Autodesk Inventor part; units mm, degrees
ref_plane "Work Plane1" through (75.8893, 0, 0) normal (0, 0.8660254, -0.5) x (-1, 0, 0)
ref_plane "YZ Plane" through (0, 0, 0) normal (1, 0, 0) x (0, 1, 0)
ref_plane "XZ Plane" through (0, 0, 0) normal (0, 1, 0) x (-1, 0, 0)
sketch "Sketch1" plane through (0, 0, 0) normal (1, 0, 0) x (0, 1, 0)
  line L0 (26.5724, 0) -> (13.2862, -23.0124)
  line L1 (13.2862, -23.0124) -> (-13.2862, -23.0124)
  line L2 (-13.2862, -23.0124) -> (-26.5724, 0)
  line L3 (-26.5724, 0) -> (-13.2862, 23.0124)
  line L4 (-13.2862, 23.0124) -> (13.2862, 23.0124)
  line L5 (13.2862, 23.0124) -> (26.5724, 0)
  point P0 (0, 0)
  point P1 (0, 0)
  dimension "d0" = 53.1449
extrude "Body" add sketch "Sketch1" along normal blind 28.575
sketch "Sketch2" plane through (0, 0, 0) normal (-1, 0, 0) x (0, 0, 1)
  point P0 (0, 0)
hole "Thread" at (0, 0, 0) direction (1, 0, 0) diameter 24.638 end through all
chamfer "Chamfer1" distance 1.964 angle 30 1 edges at (0, 0, -12.319) measured on face at (0, -16.6657, 10.0035)
chamfer "Chamfer2" distance 1.964 angle 30 1 edges at (28.575, 0, -12.319) measured on face at (28.575, -16.6657, 10.0035)
sketch "Sketch3" plane through (0, 0, 0) normal (0, 0, 1) x (1, 0, 0)
  line L0 (0, 26.5724) -> (28.575, 26.5724)
  line L1 (28.575, 13.2862) -> (28.575, 26.5724)
  line L2 (-5.715, 0) -> (34.29, 0)
  line L3 (26.9149, 26.5724) -> (28.575, 23.0124)
  dimension "d3" = 46.0248
  dimension "d4" = 25
revolve "Chamfer3" cut sketch "Sketch3" angle 360 about axis through (-10, 0, 0) along (1, 0, 0)
ref_plane "Work Plane1" through (75.8893, 0, 0) normal (0, 0.8660254, -0.5) x (-1, 0, 0)
equation "\"d0\" = 1.1547 * SW"
equation "\"d1\" = KOH"
equation "\"d3\" = SW01"
equation "\"d4\" = ANG2"
equation "\"d13\" = -0.5 * GD1 + 0.5 * NND"
equation "\"d21\" = -0.5 * GD1 + 0.5 * NND"
equation "\"d15\" = -0.5 * GD1 + 0.5 * NND"
equation "\"d22\" = -0.5 * GD1 + 0.5 * NND"
equation "\"ANG2\" = 25deg"
equation "\"NND\" = 28.575"
equation "\"KOH\" = 28.575"
equation "\"SW\" = 46.0248"
equation "\"SW01\" = SW"
equation "\"TOA\" = 30deg"
equation "\"E0\" = 1.155 * SW"
equation "\"THREADDIA\" = 28.575"
properties part number "ANSI B18.2.2 - 1 1/8 - 7, HHFNI" material "Steel, Mild"
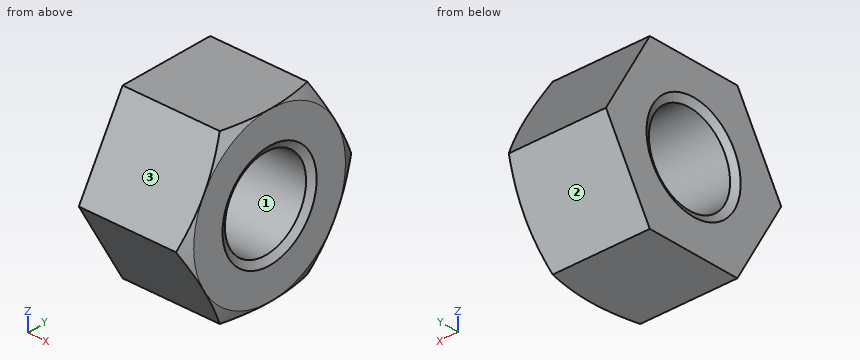
Read the model definition and answer for the solid it produces. Units are mm, in the model's axes. Face numbers are marked on the shaded views. Round coordinates to 2 decimals unless told otherwise and drop trailing zeros. Write each loop counter-clockwise with the first axis right and the second up, starting at its lowest first coordinate (ties: lowest second). Pieces come first, ordered by that corner, then holes. Notation, with made-up numbers: (28, 51.25) - (66, 51.25) arc R25 ccw to (66, 77.25) - close; hole circle Ø7 at (68.5, 70). An arc over 180 degrees is marked (long way). One line per question, with ' | ' between items. Start each with the question number.
1. Section A-A (x = 23) is taken. Determine the outline of the cut face in (y, z).
2. Find the intervals of material crossed by probe 1 along Z at (x, y) = (18, 0); probe 2 along Y at (x, z) = (13.5, 0); probe 3 along Z at (x, y) = (23.5, 9), in increasing order. Write a range as [from, to].
3. Each of these flat-tipped pins is pushed along its axis until it touches: pin 1 (5 mm diameter, centred on y = 11, z = 1.5, fed in from -X); pin 2 (6 mm diameter, centred on x = 8.5, y = 21, fed in from -Z); pin 3 (1.5 mm diameter, centred on x = 16, y = -21, fed in from +Z). Where does it stop, or does it pass through?
4. For a pull along Z with two mould halves and no side action, classify the marked faces 1, 2 and 3 as +Z half, -Z half, draft (parallel to the pull), parting line (faces both ways), or undercut.
Filled in:
1) outline: (-26.57, 0) - (-13.29, -23.01) - (13.29, -23.01) - (26.57, 0) - (13.29, 23.01) - (-13.29, 23.01) - close; hole circle Ø24.64 at (0, 0)
2) probe 1: [-23.01, -12.32], [12.32, 23.01] | probe 2: [-26.57, -12.32], [12.32, 26.57] | probe 3: [-23.01, -8.41], [8.41, 23.01]
3) pin 1: x = 0.39 | pin 2: z = -14.85 | pin 3: z = 10.95
4) face 1: undercut | face 2: -Z half | face 3: +Z half
